from build123d import *

# Parameters (mm, degrees)
SKETCH_1_R          = 10
EXTRUDE_1_DEPTH     = 10
CHAMFER_1_SIZE      = 1
CHAMFER_1_SIZE2     = 4.8
CHAMFER_2_SIZE      = 4.8
CHAMFER_2_SIZE2     = 1
SKETCH_2_R          = 3
CUT_EXTRUDE_1_DEPTH = 2.6
CUT_EXTRUDE_START   = -7.4
SKETCH_2_3_R        = 3
CUT_EXTRUDE_2_DEPTH = 2.6
SKETCH_4_R          = 1.5
CUT_EXTRUDE_3_DEPTH = 16.961202962


with BuildPart() as part:
    # 草图1 → 凸台-拉伸1 (new body)
    with BuildSketch(Plane.XY):
        Circle(SKETCH_1_R)
    extrude(amount=EXTRUDE_1_DEPTH)

    # 倒角1
    chamfer_1_edges = [part.edges().sort_by_distance(p)[0] for p in [
        (-10, 0, 0),
    ]]
    chamfer_1_side = [part.faces().sort_by_distance(p)[0] for p in [
        (0, 0, 0),
    ]]
    chamfer(chamfer_1_edges, length=CHAMFER_1_SIZE, length2=CHAMFER_1_SIZE2, reference=chamfer_1_side[0])

    # 倒角2
    chamfer_2_edges = [part.edges().sort_by_distance(p)[0] for p in [
        (-10, 0, 10),
    ]]
    chamfer_2_side = [part.faces().sort_by_distance(p)[0] for p in [
        (-10, 0, 7.4),
    ]]
    chamfer(chamfer_2_edges, length=CHAMFER_2_SIZE, length2=CHAMFER_2_SIZE2, reference=chamfer_2_side[0])

    # 草图2 → 切除-拉伸1 (cut)
    with BuildSketch(Plane(origin=(0, 0, 0), x_dir=(-1, 0, 0), z_dir=(0, 0, -1))):
        Circle(SKETCH_2_R)
    extrude(amount=-CUT_EXTRUDE_1_DEPTH, mode=Mode.SUBTRACT)

    # 草图2<3> → 切除-拉伸2 (cut)
    with BuildSketch(Plane(origin=(0, 0, 0), x_dir=(-1, 0, 0), z_dir=(0, 0, -1)).offset(CUT_EXTRUDE_START)):
        Circle(SKETCH_2_3_R)
    extrude(amount=-CUT_EXTRUDE_2_DEPTH, mode=Mode.SUBTRACT)

    # 草图4 → 切除-拉伸3 (cut, through all)
    with BuildSketch(Plane(origin=(0, 0, 2.6), x_dir=(-1, 0, 0), z_dir=(0, 0, -1))):
        Circle(SKETCH_4_R)
    extrude(amount=-CUT_EXTRUDE_3_DEPTH, mode=Mode.SUBTRACT)


solid = part.part
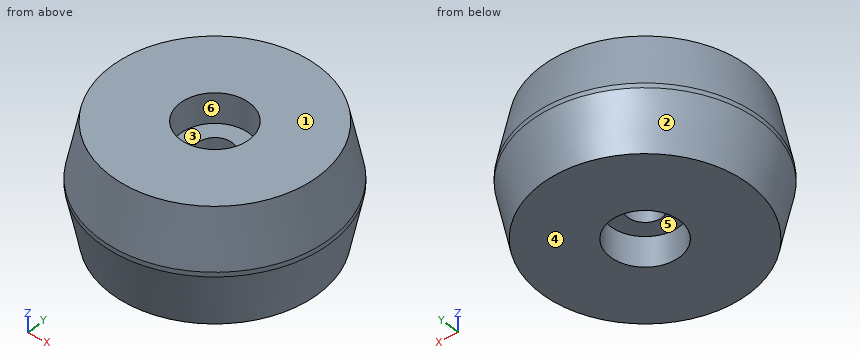
Input: part model. Units: mm. Frame: model coordinates. Face numbers are marked on the shaded views. A direction names the side the tool comes from. Round coordinates to 2 decimals unless told otherwise and drop trailing zeros. Order: outer loops, then holes, each group sorted by start corner. A loop starts at its lowest first (then second) coordinate and runs counter-clockwise, first axis right, second up. Notation, with made-up numbers: (-4.75, 71) - (9.25, 71) arc R24 ccw to (9.25, 82) - close; hole circle Ø7 at (54.5, 13). An arc over 180 degrees is marked (long way). Use a Markdown table: item, result.
1. Section C-C on z = 1.75. Return the cut outline in (x, y).
Evaluation:
| item | result |
|---|---|
| outline | circle Ø18.73 at (0, 0); hole circle Ø6 at (0, 0) |
2. Mould query, pull axis Y, two halves, no side actions, for the marked faces 1, 2 and 3. Classes: +Y half, -Y half, draft (parallel to the pull), parting line (faces both ways), or undercut.
Evaluation:
| item | result |
|---|---|
| face 1 | draft |
| face 2 | parting line |
| face 3 | undercut |
3. Section D-D on z = 4.5. Return the cut outline in (x, y) (1 decimal).
Evaluation:
| item | result |
|---|---|
| outline | circle Ø19.9 at (0, 0); hole circle Ø3 at (0, 0) |
4. Access query for the marked faces 4, 5 and 6. Directions: +Z, -Z, +X, -X, +Y, -Y. A direction counts if a zero-diameter tool reaches every point of the face in a straight line with its end or side. Return the directions, or none.
Evaluation:
| item | result |
|---|---|
| face 4 | -Z, +X, -X, +Y, -Y |
| face 5 | -Z |
| face 6 | +Z |
5. First-contact query: pin 1 (3 mm diameter, centred on x = -8, z = 9, fed in from +Y); pin 2 (1 mm diameter, centred on x = -7.5, z = 1.5, fed in from +Y); pin 3 (3 mm diameter, centred on x = 1, y = 0.5, fed in from +Z). Flat tips, straight axial feed; report the tip coordinate or a pass-through.
Evaluation:
| item | result |
|---|---|
| pin 1 | y = 6.59 |
| pin 2 | y = 6.16 |
| pin 3 | z = 7.4 |
6. Material intervals for probe 1 along Y at (x, z) = (0, 8.65); probe 2 along Y at (x, z) = (-0.5, 9); probe 3 along X at (y, z) = (2.5, 8.75), sorted ascending.
Evaluation:
| item | result |
|---|---|
| probe 1 | -9.28 to -3, 3 to 9.28 |
| probe 2 | -9.19 to -2.96, 2.96 to 9.19 |
| probe 3 | -8.92 to -1.66, 1.66 to 8.92 |
7. Section A-A on x = 0. Return the cut outline in (y, z).
Evaluation:
| item | result |
|---|---|
| outline | (-10, 4.8) - (-9, 0) - (-3, 0) - (-3, 2.6) - (-1.5, 2.6) - (-1.5, 7.4) - (-3, 7.4) - (-3, 10) - (-9, 10) - (-10, 5.2) - close; (1.5, 2.6) - (3, 2.6) - (3, 0) - (9, 0) - (10, 4.8) - (10, 5.2) - (9, 10) - (3, 10) - (3, 7.4) - (1.5, 7.4) - close |
